```python
from build123d import *

# Parameters (mm, degrees)
F1_DEPTH = 25.4
F2_T     = -2.54


with BuildPart() as f1:
    # F0 (on Front) → F1 (new body)
    with BuildSketch(Plane.XZ):
        Polygon((15.157177113, 5.0804899074), (0, 28.4029003233), (0, -45.4445231952), (10.9272608534, -26.454931125), (48.8096907386, -32.682903111), (29.9618504941, -5.8029429056), (48.8096907386, 26.9511756652), align=None)
        Polygon((0, -45.4445231952), (0, 28.4029003233), (-7.4798503051, 0), (-35.9542183578, -11.0840788111), (-3.1724292785, -18.1879308075), (-7.4798503051, -58.4431426979), align=None)
    extrude(amount=F1_DEPTH)

    # F2
    f2_openings = [f1.faces().sort_by_distance(p)[0] for p in [
        (11.533171, 0, -9.565851),
    ]]
    offset(amount=F2_T, openings=f2_openings, kind=Kind.INTERSECTION)


solid = f1.part
```
Verification items for the finished model (mm, model axes). A direction names the side the tool comes from. Round coordinates to 2 decimals unless told otherwise and drop trailing zeros. Write each loop counter-clockwise with the first axis right and the second up, starting at its lowest first coordinate (ties: lowest second). Pieces come first, ordered by that corner, then holes.
1. Section check A-A on z = 16. Enter the section's corners in (x, y).
2. Draft check along X on faces 6 (the flat face through (-5.296, -12.522, -38.034)), 7 (the flat face through (-2.015, -11.27, -31.248)), 8 (the flat face through (39.25, -12.52, 10.34)), 9 (the flat face through (34.048, -11.27, 6.391)). Enter one of: +X half, -X half, draft (parallel to the pull), parting line (faces both ways), or undercut.
3. Section check D-D on z = -7. Enter the section's corners in (x, y), plus the area to 3 significant figures.
4. Section check C-C on x = -12. Enter the section's corners in (y, z), plus the area to 3 significant figures.
5. Gauge pin test, flat ends, axial feed: P1, Ø2, axis at x = 32, y = -17.5, coming from the +Z side; P2, Ø1, axis at y = -10, z = -3.5, coming from the +X side; P3, Ø8, axis at x = 11, y = -7.5, coming from the +Z side. Record the tip position at first contact, or that the pin passes through.
6. Section check B-B on y = -9.5. Enter the section's corners in (x, z).
7. Scan lines: L1, parallel to X at y = -21.25, z = 5; L2, parallel to Z at x = 32, y = -14.75; L3, parallel to Y at x = 18, z = 1.5. Record each from-to range of solid material in increasing order.
8. Access from +Z, -Z, +X, -X, +Y, -Y to the whole of each face (thin tool, end or side, straight path). Record for faces 1 (the flat face through (13, -25.4, -8)), 2 (the flat face through (-3.688, -12.522, 14.4)), 3 (the flat face through (2.872, -11.27, -35.36)), 4 (the flat face through (7.685, -12.522, 16.578)), 5 (the flat face through (39.518, -12.522, -19.431)).
Answer:
1. outline: (-3.27, -25.4) - (8.06, -25.4) - (8.06, 0) - (5.03, 0) - (5.03, -22.86) - (-0.64, -22.86) - (-0.64, 0) - (-3.27, 0) - close; (31.96, -25.4) - (42.51, -25.4) - (42.51, 0) - (39.58, 0) - (39.58, -22.86) - (36.62, -22.86) - (36.62, 0) - (31.96, 0) - close
2. face 6: -X half
2. face 7: undercut
2. face 8: +X half
2. face 9: undercut
3. outline: (-25.46, -25.4) - (30.8, -25.4) - (30.8, 0) - (27.7, 0) - (27.7, -22.86) - (-18.46, -22.86) - (-18.46, 0) - (-25.46, 0) - close
3. area: 374 mm2
4. outline: (-25.4, -16.27) - (0, -16.27) - (0, -13.68) - (-22.86, -13.68) - (-22.86, -4.49) - (0, -4.49) - (0, -1.76) - (-25.4, -1.76) - close
4. area: 159 mm2
5. P1: stops at z = 16.68
5. P2: stops at x = 31.57
5. P3: stops at z = 17.63
6. outline: (-35.95, -11.08) - (-3.17, -18.19) - (-7.48, -58.44) - (10.93, -26.45) - (48.81, -32.68) - (29.96, -5.8) - (48.81, 26.95) - (15.16, 5.08) - (0, 28.4) - (-7.48, 0) - close; hole (-27.17, -10.39) - (-0.4, -16.19) - (-3.67, -46.73) - (9.6, -23.66) - (43.26, -29.2) - (26.95, -5.94) - (41.34, 19.07) - (14.41, 1.57) - (1, 22.21) - (-5.35, -1.9) - close
7. L1: x = -6.16 to -3.54, 12.18 to 19.69, 33.25 to 36.18
7. L2: z = -29.92 to -27.35, -13.13 to -8.71, -2.26 to 2.83, 13 to 16.03
7. L3: y = -25.4 to -22.86
8. face 1: +Z, -Z, +X, -X, -Y
8. face 2: +Z, -X, +Y, -Y
8. face 3: +Y
8. face 4: +Z, +Y, -Y
8. face 5: +X, +Y, -Y
